from build123d import *
from build123d.topology import SkipClean

# Parameters (mm, degrees)
SKETCH1_R           = 25
SKETCH1_R_2         = 23
BOSS_EXTRUDE1_DEPTH = 10
BOSS_EXTRUDE2_DEPTH = 4
BOSS_EXTRUDE3_START = 6.35
SKETCH3_R           = 25
SKETCH3_W           = 6.35
SKETCH3_H           = 6.35
BOSS_EXTRUDE3_DEPTH = 6.35


with BuildPart() as part:
    # Sketch1 → Boss-Extrude1 (new, symmetric)
    with BuildSketch(Plane(origin=(0, 0, 0), x_dir=(1, 0, 0), z_dir=(0, 1, 0))):
        with Locations(Location((0, 0, 0), (0, 0, 270))):
            Circle(SKETCH1_R)
        with Locations(Location((0, 0, 0), (0, 0, 270))):
            Circle(SKETCH1_R_2, mode=Mode.SUBTRACT)
    extrude(amount=BOSS_EXTRUDE1_DEPTH, both=True)

    # Sketch2 → Boss-Extrude2 (add)
    with SkipClean():  # the faces are left unmerged after this step: merging them gives an invalid solid
        with BuildSketch(Plane.XZ.offset(10)):
            with BuildLine():
                ThreePointArc((-1.5, 22.951034835), (0, 23), (1.5, 22.951034835))
                Line((1.5, 22.951034835), (1.5, 24.954959427))
                ThreePointArc((1.5, 24.954959427), (0.750338033, 24.98873732), (0, 25))
                ThreePointArc((0, 25), (-0.750338033, 24.98873732), (-1.5, 24.954959427))
                Line((-1.5, 24.954959427), (-1.5, 22.951034835))
            make_face()
            with BuildLine():
                Line((-24.954959427, -1.5), (-22.951034835, -1.5))
                ThreePointArc((-22.951034835, -1.5), (-23, 0), (-22.951034835, 1.5))
                Line((-22.951034835, 1.5), (-24.954959427, 1.5))
                ThreePointArc((-24.954959427, 1.5), (-24.98873732, 0.750338033), (-25, 0))
                ThreePointArc((-25, 0), (-24.98873732, -0.750338033), (-24.954959427, -1.5))
            make_face()
            with BuildLine():
                ThreePointArc((23, 0), (22.987755449, -0.750399492), (22.951034835, -1.5))
                Line((22.951034835, -1.5), (24.954959427, -1.5))
                ThreePointArc((24.954959427, -1.5), (24.98873732, -0.750338033), (25, 0))
                ThreePointArc((25, 0), (24.98873732, 0.750338033), (24.954959427, 1.5))
                Line((24.954959427, 1.5), (22.951034835, 1.5))
                ThreePointArc((22.951034835, 1.5), (22.987755449, 0.750399492), (23, 0))
            make_face()
            with BuildLine():
                Line((1.5, -24.954959427), (1.5, -22.951034835))
                ThreePointArc((1.5, -22.951034835), (0, -23), (-1.5, -22.951034835))
                Line((-1.5, -22.951034835), (-1.5, -24.954959427))
                ThreePointArc((-1.5, -24.954959427), (-0.750338033, -24.98873732), (0, -25))
                ThreePointArc((0, -25), (0.750338033, -24.98873732), (1.5, -24.954959427))
            make_face()
        extrude(amount=BOSS_EXTRUDE2_DEPTH)

    # Sketch3 → Boss-Extrude3 (add)
    with SkipClean():  # the faces are left unmerged after this step: merging them gives an invalid solid
        with BuildSketch(Plane(origin=(0, 10, 0), x_dir=(1, 0, 0), z_dir=(0, 1, 0)).offset(BOSS_EXTRUDE3_START)):
            with Locations(Location((0, 0, 0), (0, 0, 86.560187232))):
                Circle(SKETCH3_R)
            Rectangle(SKETCH3_W, SKETCH3_H, mode=Mode.SUBTRACT)
        extrude(amount=-BOSS_EXTRUDE3_DEPTH)


solid = part.part
Source: CAD feature listing. Evaluate the final solid. Frame: model axes, mm. A direction names the side the tool comes from. Give positions to 0.01 mm unless a question says otherwise; leave off trailing zeros. Loops run counter-clockwise (first coordinate to the right, second up) from the corner with the lowest first, then second, coordinate; pieces in that order, holes last. Notation, with made-up numbers: (-10.5, 4.25) -> (15.5, 4.25) arc R30 cw to (15.5, 42.25) -> close; hole circle Ø3 at (29, 25). An arc over 180 degrees is marked (long way). Use a Markdown table: item, result. Add a question column.
1) Reachability of faces 1 (the face through (17, -10, 16)), 2 (the face through (24, -12, -1.5)), 3 (the face through (0, 13, -3.175)), 4 (the face through (-1.5, -12, 24)) from +Z, -Z, +X, -X, +Y, -Y: full face, straight path, thin tool, end or side. Return the list, or none.
2) Line query: line 1 along X through (y, z) = (0.75, 0); line 2 along Y through (x, z) = (10, -9.5). Output: solid intervals per line, ascending. Write a range as [from, to].
3) Section query D-D, the plane x = -17. Return the cut outline in (y, z), then the cut area to 3 significant figures.
4) Pull-direction query (Z, two-part tool) for faces 5 (the face through (24, -12, 1.5)), 6 (the face through (0, 13, 3.175)), 7 (the face through (24, -14, 0)); classes: +Z half, -Z half, draft (parallel to the pull), parting line (faces both ways), or undercut.
5) First-contact query: pin 1 (1 mm diameter, centred on x = 24.5, y = -13, fed in from -Z); pin 2 (1 mm diameter, centred on y = -11.5, z = 24, fed in from -X); pin 3 (1.9 mm diameter, centred on y = 14, z = 0.5, fed in from +X). Flat tips, straight axial feed; report the tip coordinate or a pass-through.
6) Section query A-A, the plane y = 14. Return the cut outline in (x, z) (3 decimals).
7) Section query B-B, the plane x = 16. Return the cut outline in (y, z), then the cut area to 3 significant figures.
8) Section query C-C, the plane y = -2. Return the cut outline in (x, z).
Numbers:
| question | item | result |
|---|---|---|
| 1 | face 1 | +Z, +X, -Y |
| 1 | face 2 | -Z, +X, -X, -Y |
| 1 | face 3 | +Y, -Y |
| 1 | face 4 | +Z, -Z, -X, -Y |
| 2 | line 1 | x = [-25, -23], [23, 25] |
| 2 | line 2 | y = [10, 16.35] |
| 3 | outline | (-10, -18.33) -> (16.35, -18.33) -> (16.35, 18.33) -> (-10, 18.33) -> (-10, 15.49) -> (10, 15.49) -> (10, -15.49) -> (-10, -15.49) -> close |
| 3 | area | 346 mm2 |
| 4 | face 5 | +Z half |
| 4 | face 6 | undercut |
| 4 | face 7 | draft |
| 5 | pin 1 | stops at z = -1.5 |
| 5 | pin 2 | stops at x = -1.5 |
| 5 | pin 3 | stops at x = 25 |
| 6 | outline | circle Ø50 at (0, 0); hole (-3.175, -3.175) -> (3.175, -3.175) -> (3.175, 3.175) -> (-3.175, 3.175) -> close |
| 7 | outline | (-10, -19.21) -> (16.35, -19.21) -> (16.35, 19.21) -> (-10, 19.21) -> (-10, 16.52) -> (10, 16.52) -> (10, -16.52) -> (-10, -16.52) -> close |
| 7 | area | 351 mm2 |
| 8 | outline | circle Ø50 at (0, 0); hole circle Ø46 at (0, 0) |
